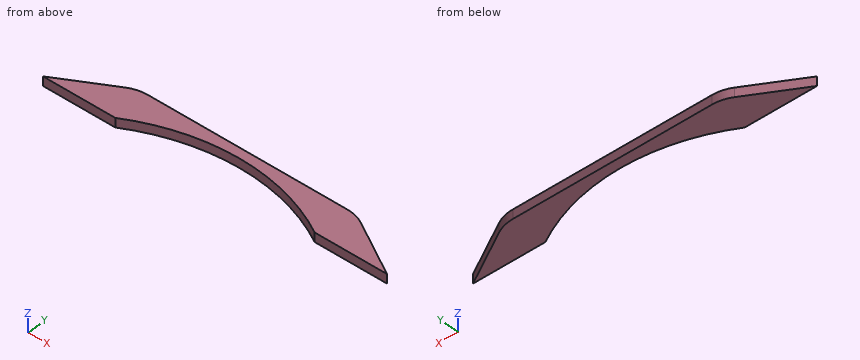
from build123d import *

# Parameters (mm, degrees)
F1_DEPTH = 5


with BuildPart() as f1:
    # F0 (on Top) → F1 (new body)
    with BuildSketch(Plane.XY):
        Polygon((-92.8162193303, -9.75), (-53.8162193302, -9.75), (-63.5662193303, 7.1374953738), align=None)
        with BuildLine():
            Line((-63.5662193303, 7.1374953738), (-53.8162193303, -9.75))
            Line((-53.8162193303, -9.75), (-53.8162193303, 9.75))
            ThreePointArc((-53.8162193303, 9.75), (-58.8631907097, 9.0855536126), (-63.5662193303, 7.1374953738))
        make_face()
        with BuildLine():
            Line((-53.8162193303, 9.75), (-53.8162193303, -9.75))
            ThreePointArc((-53.8162193303, -9.75), (-53.3700027957, 0.0405892766), (-52.0350529909, 9.75))
            Line((-52.0350529909, 9.75), (-53.8162193303, 9.75))
        make_face()
        with BuildLine():
            ThreePointArc((-53.8162193302, -9.75), (0, 4.6700125092), (53.8162193302, -9.75))
            ThreePointArc((53.8162193303, -9.75), (53.3700027957, 0.0405892766), (52.0350529909, 9.75))
            Line((52.0350529909, 9.75), (-52.0350529909, 9.75))
            ThreePointArc((-52.0350529909, 9.75), (-53.3700027957, 0.0405892766), (-53.8162193303, -9.75))
        make_face()
        with BuildLine():
            ThreePointArc((52.0350529909, 9.75), (53.3700027957, 0.0405892766), (53.8162193303, -9.75))
            Line((53.8162193303, -9.75), (53.8162193303, 9.75))
            Line((53.8162193303, 9.75), (52.0350529909, 9.75))
        make_face()
        with BuildLine():
            Line((53.8162193303, 9.75), (53.8162193303, -9.75))
            Line((53.8162193303, -9.75), (63.5662193303, 7.1374953738))
            ThreePointArc((63.5662193303, 7.1374953738), (58.8631907097, 9.0855536126), (53.8162193303, 9.75))
        make_face()
        Polygon((63.5662193303, 7.1374953738), (53.8162193303, -9.75), (92.8162193303, -9.75), align=None)
    extrude(amount=F1_DEPTH)


solid = f1.part
For this review, take the finished solid that the model builds, in its own axes (mm). Round coordinates to 2 decimals unless told otherwise and drop trailing zeros. Write each loop counter-clockwise with the first axis right and the second up, starting at its lowest first coordinate (ties: lowest second). Pieces come first, ordered by that corner, then holes. Notation, with made-up numbers: (70, 86.25) - (114, 86.25) arc R30 cw to (114, 120.25) - close; hole circle Ø5 at (83.25, -17). An arc over 180 degrees is marked (long way). Write item = value, one per line. Start each with the question number.
1. Wall thickness on L1, parallel to X at y = -7.5, z = 3.6; L2, parallel to X at y = -6.75, z = 1.55; L3, parallel to Y at x = 9, z = 1.1: over which ranges is each line inside the solid? List them lowest first.
2. Consider section D-D on x = -31. State the section outline as (y, z) points.
3. Consider section C-C on y = -7.25. State the section outline as (x, z) points, plus the area to 3 significant figures.
4. Consider section A-A on y = 3. State the section outline as (x, z) points.
5. Consider section B-B on z = 1.4. State the section outline as (x, y) points.
Evaluation:
q1.L1 = -88.92 to -49.72, 49.72 to 88.92
q1.L2 = -87.62 to -48.25, 48.25 to 87.62
q1.L3 = 4.29 to 9.75
q2.outline = (0.11, 0) - (9.75, 0) - (9.75, 5) - (0.11, 5) - close
q3.outline = (-88.49, 0) - (-49.23, 0) - (-49.23, 5) - (-88.49, 5) - close; (49.23, 0) - (88.49, 0) - (88.49, 5) - (49.23, 5) - close
q3.area = 393 mm2
q4.outline = (-70.73, 0) - (-18.89, 0) - (-18.89, 5) - (-70.73, 5) - close; (18.89, 0) - (70.73, 0) - (70.73, 5) - (18.89, 5) - close
q5.outline = (-92.82, -9.75) - (-53.82, -9.75) arc R107.63 cw to (53.82, -9.75) - (92.82, -9.75) - (63.57, 7.14) arc R19.5 ccw to (53.82, 9.75) - (-53.82, 9.75) arc R19.5 ccw to (-63.57, 7.14) - close
